Part model, mm, in its own coordinate system. A direction names the side the tool comes from. Round coordinates to 2 decimals unless told otherwise and drop trailing zeros. Write each loop counter-clockwise with the first axis right and the second up, starting at its lowest first coordinate (ties: lowest second). Pieces come first, ordered by that corner, then holes. Notation, with made-up numbers: M 79,80.25 L 96,80.25 A19 ccw 96,117.25 Z; hole C 11.25,85.25 d8. An arc over 180 degrees is marked long. Answer as a JSON object with one key per item and string values. Group by question number.
1. Two-plate mould, pull along X, no slides. Class faces 1 (the face through (-79.373, 3.493, 29.58)), 2 (the face through (-1, -17, 0)), 3 (the face through (-1, -16, 5)): +X half, -X half, draft (parallel to the pull), parting line (faces both ways), or undercut.
2. Band-saw the part on C-C, the plane x = 35. Write the cut outline in (y, z).
3. Which spindle directions (+Z, -Z, +X, -X, +Y, -Y) get a long thin tool onto all of the face, cutting with end or side? Do faces 4 (the face through (71, 22.4, 32.1)), 5 (the face through (-9.851, 0, 2)), 6 (the face through (-71, -23, 60)). Say none if no direction does.
4. Band-saw the part on A-A, the plane x = 0. Write the cut outline in (y, z), plus the area to 3 significant figures.
5. Band-saw the part on D-D, the plane z = 42. Write the cut outline in (x, y), plus the area to 3 significant figures.
6. Drop flat-ended pins along their axis: pin 1 (2 mm diameter, centred on y = -57, z = 23, fed in from -X); pin 2 (1.5 mm diameter, centred on x = 1.5, z = 1.5, fed in from +Y); pin 3 (5.5 mm diameter, centred on x = 10, z = 2.5, fed in from -Y). Give the stop position or say it passes through.
7. Drill centre lines: line 1 (X direction, y = 1, z = 18); line 2 (Y direction, x = 32, z = 47.5); line 3 (X direction, y = -22, z = 46.5). Where is each one in solid material? Low to high. Write a range as from..to.
8. Band-saw the part on B-B, the plane y = 0. Write the cut outline in (x, z).
from build123d import *

# Parameters (mm, degrees)
SKETCH1_R           = 79.45
BOSS_EXTRUDE1_DEPTH = 60
SHELL1_T            = -5
SKETCH2_R           = 2.5
CUT_EXTRUDE1_DEPTH  = 60
SKETCH3_R           = 2.1
CUT_EXTRUDE2_DEPTH  = 60


with BuildPart() as part:
    # Sketch1 → Boss-Extrude1 (new body)
    with BuildSketch(Plane.XY):
        Circle(SKETCH1_R)
    extrude(amount=BOSS_EXTRUDE1_DEPTH)

    # Shell1
    shell1_openings = [part.faces().sort_by_distance(p)[0] for p in [
        (0, 0, 60),
    ]]
    offset(amount=SHELL1_T, openings=shell1_openings, kind=Kind.INTERSECTION)

    # Sketch2 → Cut-Extrude1 (cut)
    with BuildSketch(Plane.XY.offset(5)):
        Circle(SKETCH2_R)
    extrude(amount=-CUT_EXTRUDE1_DEPTH, mode=Mode.SUBTRACT)

    # Sketch3 → Cut-Extrude2 (cut)
    with BuildSketch(Plane(origin=(0, 0, 0), x_dir=(-1, 0, 0), z_dir=(0, 0, -1))):
        with Locations((-34.810395013, 4.930302556)):
            Circle(SKETCH3_R)
        with Locations((-34.811895415, -4.91969733)):
            Circle(SKETCH3_R)
        with Locations((14.610395247, -4.927225588)):
            Circle(SKETCH3_R)
        with Locations((14.61189565, 4.922774298)):
            Circle(SKETCH3_R)
        Polygon((-30.048499249, 9.854577256), (9.851454591, 9.84849949), (9.851454591, -9.851500739), (-30.051500054, -9.845422515), align=None)
    extrude(amount=-CUT_EXTRUDE2_DEPTH, mode=Mode.SUBTRACT)


solid = part.part
Worked answers:
{
 "1": {"face 1": "parting line", "face 2": "draft", "face 3": "undercut"},
 "2": {"outline": "M -71.33,0 L -7.01,0 L -7.01,5 L -65.71,5 L -65.71,60 L -71.33,60 Z; M -2.83,0 L 2.84,0 L 2.84,5 L -2.83,5 Z; M 7.02,0 L 71.33,0 L 71.33,60 L 65.71,60 L 65.71,5 L 7.02,5 Z"},
 "3": {"face 4": "+Z", "face 5": "+Z, -Z", "face 6": "+Z, +X, -X, +Y, -Y"},
 "4": {"outline": "M -79.45,0 L -9.85,0 L -9.85,5 L -74.45,5 L -74.45,60 L -79.45,60 Z; M 9.85,0 L 79.45,0 L 79.45,60 L 74.45,60 L 74.45,5 L 9.85,5 Z", "area": "1,250 mm^2"},
 "5": {"outline": "C 0,0 d158.9; hole C 0,0 d148.9", "area": "2,420 mm^2"},
 "6": {"pin 1": "stops at x = -56.36", "pin 2": "stops at y = 79.45", "pin 3": "stops at y = -79.12"},
 "7": {"line 1": "x = -79.44..-74.44, 74.44..79.44", "line 2": "y = -72.72..-67.22, 67.22..72.72", "line 3": "x = -76.34..-71.13, 71.13..76.34"},
 "8": {"outline": "M -79.45,0 L -9.85,0 L -9.85,5 L -74.45,5 L -74.45,60 L -79.45,60 Z; M 30.05,0 L 79.45,0 L 79.45,60 L 74.45,60 L 74.45,5 L 30.05,5 Z"}
}
